Autodesk Inventor part; units mm, degrees
ref_plane "YZ Plane" through (0, 0, 0) normal (1, 0, 0) x (0, 1, 0)
ref_plane "XZ Plane" through (0, 0, 0) normal (0, 1, 0) x (-1, 0, 0)
ref_plane "XY Plane" through (0, 0, 0) normal (0, 0, 1) x (1, 0, 0)
sketch "Boceto1" plane through (0, 0, 0) normal (1, 0, 0) x (0, 1, 0)
  line L0 (27, 0) -> (0, 0)
  line L1 (0, 0) -> (0, 6.55)
  line L2 (0, 6.55) -> (27, 6.55)
  line L3 (27, 6.55) -> (27, 0)
  line L4 (0, 6.55) -> (5, 6.55)
  line L5 (5, 6.55) -> (5, 21.55)
  line L6 (5, 21.55) -> (0, 21.55)
  line L7 (0, 21.55) -> (0, 6.55)
  dimension "d0" = 27
  dimension "d1" = 6.55
  dimension "d2" = 15
  dimension "d3" = 5
extrude "Extrusión1" add sketch "Boceto1" along normal mid plane 17.8
sketch "Boceto3" plane through (8.9, 27, 0) normal (0, 0, -1) x (-1, 0, 0)
  line L0 (4.9, -19) -> (12.9, -19)
  line L1 (12.9, -19) -> (12.9, -27)
  line L2 (12.9, -27) -> (4.9, -27)
  line L3 (4.9, -27) -> (4.9, -19)
  line L4 (0, -27) -> (17.8, -27)
  point P0 (8.9, -27)
  point P1 (8.9, -27)
  dimension "d6" = 8
  dimension "d7" = 8
extrude "Extrusión2" cut sketch "Boceto3" against normal through all
sketch "Boceto4" plane through (-8.9, 5, 21.55) normal (0, 1, 0) x (1, 0, 0)
  point P0 (8.9, 21.55)
sketch "Boceto5" plane through (-8.9, 27, 6.55) normal (0, 1, 0) x (1, 0, 0)
  circle A0 centre (3.8, 3.1) radius 2
  circle A1 centre (14, 3.1) radius 2
  line L0 (0, 0) -> (0, 6.55)
  line L1 (0, 0) -> (17.8, 0)
  line L2 (17.8, 6.55) -> (17.8, 0)
  point P0 (8.9, 6.55)
  dimension "d10" = 4
  dimension "d11" = 4
  dimension "d12" = 3.8
  dimension "d13" = 3.1
  dimension "d14" = 3.8
extrude "Extrusión3" cut sketch "Boceto5" against normal blind 10
sketch "Boceto6" plane through (-8.9, 5, 21.55) normal (0, 1, 0) x (1, 0, 0)
  circle A0 centre (2.45, 7.5) radius 1.75
  circle A1 centre (15.35, 7.5) radius 1.75
  line L0 (0, 0) -> (4.9, 0)
  line L1 (0, 15) -> (17.8, 15)
  line L2 (12.9, 0) -> (17.8, 0)
  point P0 (8.9, 21.55)
  point P1 (2.45, 0)
  point P2 (15.35, 0)
  dimension "d17" = 3.5
  dimension "d18" = 3.5
  dimension "d19" = 15
  dimension "d20" = 7.5
  dimension "d21" = 7.5
extrude "Extrusión4" cut sketch "Boceto6" against normal through all
fillet "Empalme1" radius 2 2 edges at (-6.45, 5, 6.55) (6.45, 5, 6.55)
fillet "Empalme2" radius 2 2 edges at (-6.45, 5, 21.55) (6.45, 5, 21.55)
move faces "Desplazar1" translate (0, 2, 0) faces at (1.6196, 27, 0.4882)
equation "\"d11\" = d10"
equation "\"d14\" = d12"
equation "\"d20\" = 0.5 * d19"
equation "\"d21\" = d20"
properties part number "Sujeción de servo a mesa" material "Plástico PC/ABS"
Geometry: final body of the model. Coordinates: model frame, mm. A direction names the side the tool comes from. Coordinates: 2 decimals unless noted, no trailing zeros. Loops run counter-clockwise (first coordinate to the right, second up) from the corner with the lowest first, then second, coordinate; pieces in that order, holes last. Notation, with made-up numbers: (14.25, 17.5) -> (34.25, 17.5) arc R9 ccw to (34.25, 29.5) -> close; hole circle Ø3 at (-35, -13). An arc over 180 degrees is marked (long way). Use a Markdown table: item, result. Add a question column.
(1) Access query for faces 1 (the flat face through (-5, 17, 3)), 2 (the flat face through (0, 18, 6.55)), 3 (the cylindrical face through (-7.84, 2.54, 15.11)), 4 (the flat face through (0, 8, 3)). Directions: +Z, -Z, +X, -X, +Y, -Y. A direction counts if a zero-diameter tool reaches every point of the face in a straight line with its end or side. Return the directions, or none.
(2) Section query B-B, the plane x = 6.5. Return loops of the section in (y, z), plus the area to 3 significant figures.
(3) Section query A-A, the plane y = 3.5. Return loops of the section in (x, z), plus the area to 3 significant figures.
(4) Section query C-C, the plane y = 25.75. Return loops of the section in (x, z).
(5) Mould query, pull axis X, two halves, no side actions, for faces 5 (the flat face through (-6, 0, 11)), 6 (the flat face through (-8.9, 11, 6)), 7 (the cylindrical face through (6.947, 23.084, 4.216)), 8 (the flat face through (8.9, 11, 6)). Classes: pulls with the +X half, pulls with the -X half, needs draft (parallel to the pull), parting line crosses it, or undercut.
(6) Line query: line 1 along X through (y, z) = (26.25, 3.45); line 2 along Z through (x, y) = (-5.1, 20.5); line 3 along Z through (x, y) = (-6.45, 1.4). Output: solid intervals per line, ascending.
(7) Pin query (flat end, axial travel): pin 1 Ø1.5 at (x, z) = (7, 15) entering from +Y; pin 2 Ø5 at (x, z) = (-0.5, 3.5) entering from -Y; pin 3 Ø2.5 at (x, z) = (-5.1, 3.45) entering from +Y. Return the tip coordinate at first contact, or that it passes through.
(8) Section query D-D, the plane z = 2.5. Return loops of the section in (x, y), plus the area to 3 significant figures.
Answer:
| question | item | result |
|---|---|---|
| 1 | face 1 | +Y |
| 1 | face 2 | +Z, +X, -X, +Y |
| 1 | face 3 | +Y, -Y |
| 1 | face 4 | +Z, -Z, -Y |
| 2 | outline | (0, 0) -> (29, 0) -> (29, 2.02) -> (17, 2.02) -> (17, 4.88) -> (29, 4.88) -> (29, 6.55) -> (7, 6.55) arc R2 cw to (5, 8.55) -> (5, 12.3) -> (0, 12.3) -> close; (0, 15.8) -> (5, 15.8) -> (5, 19.55) arc R2 ccw to (3, 21.55) -> (0, 21.55) -> close |
| 2 | area | 213 mm^2 |
| 3 | outline | (-8.9, 0) -> (-4, 0) -> (-4, 21.49) -> (-8.9, 21.49) -> close; (4, 0) -> (8.9, 0) -> (8.9, 21.49) -> (4, 21.49) -> close; hole circle Ø3.5 at (-6.45, 14.05); hole circle Ø3.5 at (6.45, 14.05) |
| 3 | area | 191 mm^2 |
| 4 | outline | (-8.9, 0) -> (8.9, 0) -> (8.9, 6.55) -> (-8.9, 6.55) -> close; hole circle Ø4 at (-5.1, 3.45); hole circle Ø4 at (5.1, 3.45) |
| 5 | face 5 | needs draft |
| 5 | face 6 | pulls with the -X half |
| 5 | face 7 | undercut |
| 5 | face 8 | pulls with the +X half |
| 6 | line 1 | x = -8.9 to -7.1, -3.1 to 3.1, 7.1 to 8.9 |
| 6 | line 2 | z = 0 to 1.45, 5.45 to 6.55 |
| 6 | line 3 | z = 0 to 12.3, 15.8 to 21.55 |
| 7 | pin 1 | stops at y = 5 |
| 7 | pin 2 | stops at y = 8 |
| 7 | pin 3 | stops at y = 17 |
| 8 | outline | (-8.9, 0) -> (-4, 0) -> (-4, 8) -> (4, 8) -> (4, 0) -> (8.9, 0) -> (8.9, 29) -> (6.86, 29) -> (6.86, 17) -> (3.34, 17) -> (3.34, 29) -> (-3.34, 29) -> (-3.34, 17) -> (-6.86, 17) -> (-6.86, 29) -> (-8.9, 29) -> close |
| 8 | area | 368 mm^2 |
